Source: CAD feature listing. Evaluate the final solid. Frame: model axes, mm. A direction names the side the tool comes from. Give positions to 0.01 mm unless a question says otherwise; leave off trailing zeros. Order: outer loops, then holes, each group sorted by start corner. A loop starts at its lowest first (then second) coordinate and runs counter-clockwise, first axis right, second up. Notation, with made-up numbers: (76.5, -6) -> (130.5, -6) arc R22 cw to (130.5, 7) -> close; hole circle Ø11 at (68.25, 88). An arc over 180 degrees is marked (long way). Use CSV: the item, a comma, the result in double quotes.
```python
from build123d import *

# Parameters (mm, degrees)
F3_DEPTH  = 4.9
F4_R      = 20
F4_R_2    = 4
F5_DEPTH  = 4.9
F6_DEPTH  = 8
F7_R      = 5
F9_D      = 5.43
F9_DEPTH  = 1.1
F9_TIP    = 1.6313365807
F10_D     = 5.43
F10_DEPTH = 2.2
F10_TIP   = 1.6313365807
F11_R     = 10.5
F12_DEPTH = 100
F14_DEPTH = 5


with BuildPart() as f2:
    # F0 (on Front) → F2 (revolve)
    with BuildSketch(Plane.XZ):
        with BuildLine():
            Line((4, 0), (25, 0))
            ThreePointArc((25, 0), (25.0633115181, 44.8380443487), (45, 85))
            Line((45, 85), (10, 85))
            ThreePointArc((10, 85), (5.5209994492, 72.8549601322), (4, 60))
            Line((4, 60), (4, 0))
        make_face()
    revolve(axis=Axis((0, 0, 25.1682717353), (0, 0, 1)))

    # F3 (add): a face of the model
    f3_faces = [f2.faces().sort_by_distance(p)[0] for p in [
        (-4.7071067812, 0, 0),
    ]]
    extrude(f3_faces, amount=F3_DEPTH)

    # F4 (on face) → F5 (cut)
    with BuildSketch(Plane(origin=(0, 0, -4.9), x_dir=(1, 0, 0), z_dir=(0, 0, -1))):
        Circle(F4_R)
        Circle(F4_R_2, mode=Mode.SUBTRACT)
    extrude(amount=-F5_DEPTH, mode=Mode.SUBTRACT)

    # F6 (add): a face of the model
    f6_faces = [f2.faces().sort_by_distance(p)[0] for p in [
        (-43.7272077939, 0, 85),
    ]]
    extrude(f6_faces, amount=F6_DEPTH)

    # F7
    f7_edges = [f2.edges().sort_by_distance(p)[0] for p in [
        (-45, 0, 93),
    ]]
    fillet(f7_edges, radius=F7_R)

    # F9
    with Locations(Plane.XY.offset(93)):
        with Locations((14.426644952, 0.1037907432), (-14.573297048, 0)):
            Hole(F9_D / 2, depth=F9_DEPTH)
            with Locations((0, 0, -(F9_DEPTH + F9_TIP / 2))):  # 118° drill point
                Cone(0, F9_D / 2, F9_TIP, mode=Mode.SUBTRACT)

    # F10
    with Locations(Plane.XY.offset(93)):
        with Locations((0, -20.4359735063)):
            Hole(F10_D / 2, depth=F10_DEPTH)
            with Locations((0, 0, -(F10_DEPTH + F10_TIP / 2))):  # 118° drill point
                Cone(0, F10_D / 2, F10_TIP, mode=Mode.SUBTRACT)

    # F11 (on Top) → F12 (cut)
    with BuildSketch(Plane.XY):
        Circle(F11_R)
    extrude(amount=F12_DEPTH, mode=Mode.SUBTRACT)

    # F13 (on face) → F14 (join)
    with BuildSketch(Plane(origin=(0, 0, -4.9), x_dir=(1, 0, 0), z_dir=(0, 0, -1))):
        with BuildLine():
            ThreePointArc((2.125, -24.9095237811), (0, -25), (-2.125, -24.9095237811))
            Line((-2.125, -24.9095237811), (-2.125, -26.9095237811))
            Line((-2.125, -26.9095237811), (2.125, -26.9095237811))
            Line((2.125, -26.9095237811), (2.125, -24.9095237811))
        make_face()
    extrude(amount=-F14_DEPTH)


solid = f2.part
```
1. Ray query, line 1 along Y through (x, z) = (0, -1); line 2 along X through (y, z) = (0, -1); line 3 along Y through (x, z) = (0, 92). Return the intervals inside material, ascending.
Answer below:
line 1,"y = -25 to -20, 20 to 26.91"
line 2,"x = -25 to -20, 20 to 25"
line 3,"y = -43 to -23.15, -17.72 to -10.5, 10.5 to 43"
2. Section query A-A on z = 40.5. Return loops of the section in (x, y).
Answer below:
outline,"circle Ø48.29 at (0, 0); hole circle Ø21 at (0, 0)"
3. Access query for faces 1 (the flat face through (8, -8, 93)), 2 (the cylindrical face through (17.14, 0.22, 92.44)), 3 (the flat face through (9, 9, 0)). Directions: +Z, -Z, +X, -X, +Y, -Y. A direction counts if a zero-diameter tool reaches every point of the face in a straight line with its end or side. Return the directions, or none.
Answer below:
face 1,"+Z, +X, -X, +Y, -Y"
face 2,"+Z"
face 3,"-Z"
4. Section query B-B on z = 14. Return loops of the section in (x, y).
Answer below:
outline,"circle Ø45.59 at (0, 0); hole circle Ø21 at (0, 0)"
5. Mould query, pull axis Y, two halves, no side actions, for faces 4 (the flat face through (0, 26.91, -2)), 5 (the conical face through (14.05, -0.18, 90.55)), 6 (the cylindrical face through (-9.76, -43.93, 86.48)), 7 (the flat face through (-0.1, -20.3, -4.9)). Classes: released by +Y, released by -Y, zero draft, split by the parting line, or undercut.
Answer below:
face 4,"released by +Y"
face 5,"undercut"
face 6,"split by the parting line"
face 7,"zero draft"
6. Pin query (flat end, axial travel): P1, Ø4, axis at x = -6.5, z = 10, coming from the -Y side; P2, Ø10, axis at x = 33.5, y = -32.5, coming from the -Z side; P3, Ø1.6, axis at y = 26, z = -3, coming from the +X side (3 decimals). Return the tip coordinate at first contact, or that it passes through.
Answer below:
P1,"stops at y = -22.85"
P2,"stops at z = 80.74"
P3,"stops at x = 2.125"
